Input: part model. Units: mm. Frame: model coordinates. A direction names the side the tool comes from. Coordinates: 2 decimals unless noted, no trailing zeros. Order: outer loops, then holes, each group sorted by start corner. A loop starts at its lowest first (then second) coordinate and runs counter-clockwise, first axis right, second up. Notation, with made-up numbers: (62.5, 57) - (118.5, 57) arc R17 cw to (118.5, 86) - close; hole circle Ø1 at (60, -30). An arc over 180 degrees is marked (long way). One line per question, with ' | ' between items.
from build123d import *

# Parameters (mm, degrees)
SKETCH_1_W          = 46
SKETCH_1_H          = 14
EXTRUDE_1_DEPTH     = 7
CUT_EXTRUDE_1_REACH = 27.04
SKETCH_2_R          = 1.5
CUT_EXTRUDE_2_REACH = 29.821
SKETCH_3_R          = 3.65
SKETCH_4_R          = 3
CUT_EXTRUDE_3_DEPTH = 3.8
FILLET_1_R          = 5


with BuildPart() as part:
    # Эскиз1 → Бобышка-Вытянуть1 (new body)
    with BuildSketch(Plane.XY):
        Rectangle(SKETCH_1_W, SKETCH_1_H)
    extrude(amount=EXTRUDE_1_DEPTH)

    # Эскиз2 → Вырез-Вытянуть1 (cut, up to next)
    with BuildSketch(Plane.XY.offset(7), mode=Mode.PRIVATE) as cut_extrude_1_sk1:
        with Locations((-8, 0)):
            Circle(SKETCH_2_R)
    cut_extrude_1_tool1 = extrude(cut_extrude_1_sk1.sketch, amount=-CUT_EXTRUDE_1_REACH, mode=Mode.PRIVATE) & part.part
    # Эскиз2 → Вырез-Вытянуть1 (cut, up to next)
    with BuildSketch(Plane.XY.offset(7), mode=Mode.PRIVATE) as cut_extrude_1_sk2:
        with Locations(Location((8, 0, 0), (0, 0, 180))):
            Circle(SKETCH_2_R)
    cut_extrude_1_tool2 = extrude(cut_extrude_1_sk2.sketch, amount=-CUT_EXTRUDE_1_REACH, mode=Mode.PRIVATE) & part.part
    add(cut_extrude_1_tool1.solids().sort_by_distance((-8, 0, 7))[0], mode=Mode.SUBTRACT)
    add(cut_extrude_1_tool2.solids().sort_by_distance((8, 0, 7))[0], mode=Mode.SUBTRACT)

    # Эскиз3 → Вырез-Вытянуть2 (cut, up to next)
    with BuildSketch(Plane(origin=(0, 7, 0), x_dir=(1, 0, 0), z_dir=(0, 1, 0)), mode=Mode.PRIVATE) as cut_extrude_2_sk1:
        with Locations((-15, -7.5)):
            Circle(SKETCH_3_R)
    cut_extrude_2_tool1 = extrude(cut_extrude_2_sk1.sketch, amount=-CUT_EXTRUDE_2_REACH, mode=Mode.PRIVATE) & part.part
    # Эскиз3 → Вырез-Вытянуть2 (cut, up to next)
    with BuildSketch(Plane(origin=(0, 7, 0), x_dir=(1, 0, 0), z_dir=(0, 1, 0)), mode=Mode.PRIVATE) as cut_extrude_2_sk2:
        with Locations((15, -7.5)):
            Circle(SKETCH_3_R)
    cut_extrude_2_tool2 = extrude(cut_extrude_2_sk2.sketch, amount=-CUT_EXTRUDE_2_REACH, mode=Mode.PRIVATE) & part.part
    add(cut_extrude_2_tool1.solids().sort_by_distance((-15, 7, 7.5))[0], mode=Mode.SUBTRACT)
    add(cut_extrude_2_tool2.solids().sort_by_distance((15, 7, 7.5))[0], mode=Mode.SUBTRACT)

    # Эскиз4 → Вырез-Вытянуть3 (cut)
    with BuildSketch(Plane(origin=(0, 0, 0), x_dir=(-1, 0, 0), z_dir=(0, 0, -1))):
        with Locations((-8, 0)):
            Circle(SKETCH_4_R)
        with Locations((8, 0)):
            Circle(SKETCH_4_R)
    extrude(amount=-CUT_EXTRUDE_3_DEPTH, mode=Mode.SUBTRACT)

    # Скругление1
    fillet_1_edges = [part.edges().sort_by_distance(p)[0] for p in [
        (-23, 0, 0),
        (23, 0, 0),
    ]]
    fillet(fillet_1_edges, radius=FILLET_1_R)


solid = part.part
Item 1: Ray query, line 1 (Y direction, x = 8, z = 2.25); line 2 (Y direction, x = 8, z = 4.8); line 3 (X direction, y = -5.5, z = 5.25). Return the intervals inside material, ascending.
Data:
line 1: -7 to -3, 3 to 7 | line 2: -7 to -1.5, 1.5 to 7 | line 3: -23 to -17.87, -12.13 to 12.13, 17.87 to 23
Item 2: Section D-D on z = 1.5. Return the cut outline in (x, y).
Data:
outline: (-21.57, -7) - (21.57, -7) - (21.57, 7) - (-21.57, 7) - close; hole circle Ø6 at (-8, 0); hole circle Ø6 at (8, 0)
Item 3: Draft query along X for faces 3 (the face through (0, 7, 3)), 4 (the face through (5.23, -1.15, 1.87)), 5 (the face through (-23, 0, 6)). Return one class per face: released by +X, released by -X, zero draft, split by the parting line, or undercut.
Data:
face 3: zero draft | face 4: undercut | face 5: released by -X
Item 4: Contact query for flat-ended pins moving along their axis: P1, Ø3, axis at x = 14, y = -5, coming from the +Z side; P2, Ø1.5, axis at x = -13.5, y = 2.5, coming from the +Z side. Output: stop coordinate, or through.
Data:
P1: z = 4.84 | P2: z = 4.63
Item 5: Section A-A on x = -8. Return the cut outline in (y, z).
Data:
outline: (-7, 0) - (-3, 0) - (-3, 3.8) - (-1.5, 3.8) - (-1.5, 7) - (-7, 7) - close; (1.5, 3.8) - (3, 3.8) - (3, 0) - (7, 0) - (7, 7) - (1.5, 7) - close
Item 6: Section B-B on y = 0. Return the cut outline in (x, z).
Data:
outline: (-23, 5) arc R5 ccw to (-18, 0) - (-11, 0) - (-11, 3.8) - (-9.5, 3.8) - (-9.5, 7) - (-11.38, 7) arc R3.65 cw to (-18.62, 7) - (-23, 7) - close; (-6.5, 3.8) - (-5, 3.8) - (-5, 0) - (5, 0) - (5, 3.8) - (6.5, 3.8) - (6.5, 7) - (-6.5, 7) - close; (9.5, 3.8) - (11, 3.8) - (11, 0) - (18, 0) arc R5 ccw to (23, 5) - (23, 7) - (18.62, 7) arc R3.65 cw to (11.38, 7) - (9.5, 7) - close
Item 7: Section C-C on y = -3.5. Return the cut outline in (x, z), and give its area (3 significant figures).
Data:
outline: (-23, 5) arc R5 ccw to (-18, 0) - (18, 0) arc R5 ccw to (23, 5) - (23, 7) - (18.62, 7) arc R3.65 cw to (11.38, 7) - (-11.38, 7) arc R3.65 cw to (-18.62, 7) - (-23, 7) - close | area: 277 mm^2
Item 8: Access query for faces 1 (the face through (6.7, -1.3, 3.8)), 2 (the face through (21, 0, 1)). Directions: +Z, -Z, +X, -X, +Y, -Y. A direction counts if a zero-diameter tool reaches every point of the face in a straight line with its end or side. Return the directions, or none.
Data:
face 1: -Z | face 2: -Z, +X, +Y, -Y
